Print and shaded views of the part. All mm, measured from the part's lowest x, y and z. A direction names the side the tool comes from. Round coordinates to 2 decimals unless told otherwise and drop trailing zeros. Write each loop counter-clockwise with the first axis right and the second up, starting at its lowest first coordinate (ties: lowest second). Pieces come first, ordered by that corner, then holes. Notation, with made-up numbers: (0.25, 30) - (44.25, 30) arc R19 ccw to (44.25, 59) - close; hole circle Ø9 at (66, 31.25). An arc over 180 degrees is marked (long way). Answer as a JSON object with one key per item and string values. Group by question number.
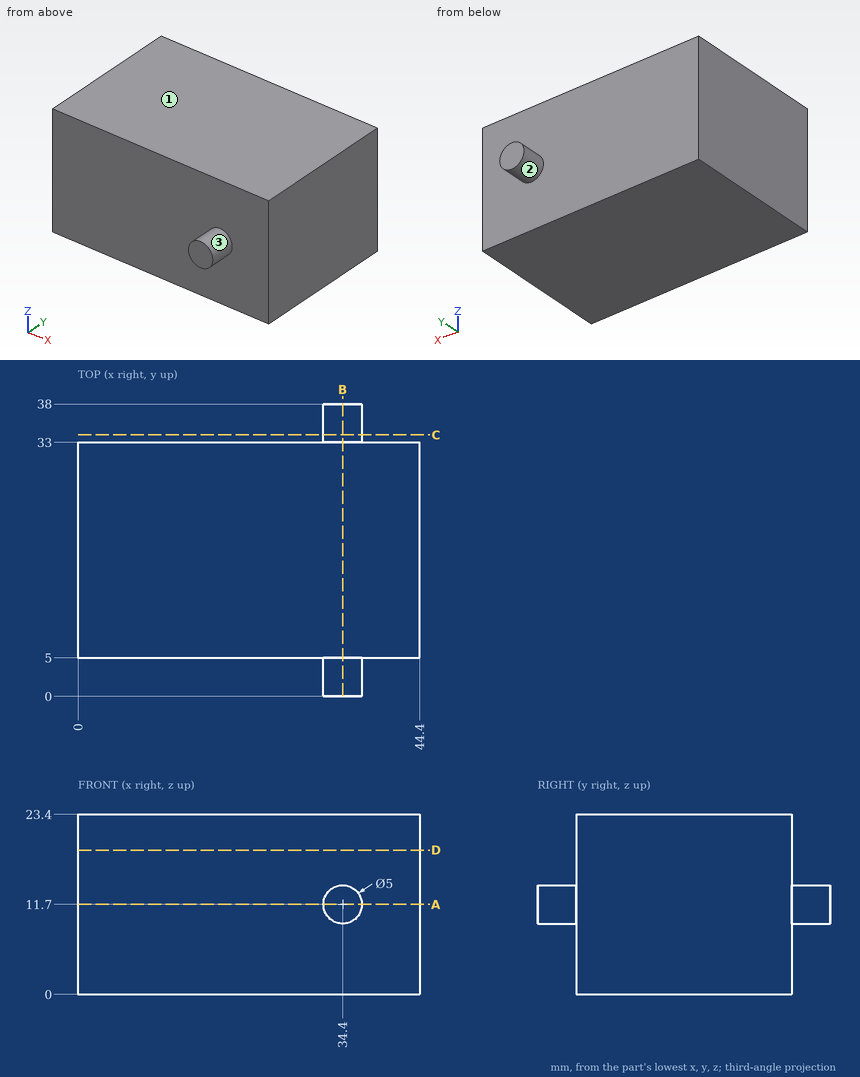
(1) Flat gauge pins, fed straight in: pin 1 (7 mm diameter, centred on x = 11, z = 11, fed in from -Y); pin 2 (6 mm diameter, centred on x = 12.5, z = 9.5, fed in from +Y). Where does each tip first touch, or does it go through?
(2) 3-axis set-ups, long thin cutter, end or side, ignore diameter. For the marked faces 1, 2 and 3: which of +Z, -Z, +X, -X, +Y, -Y reach the whole face in a straight line?
(3) Slice it at D-D (z = 18.75). Write the cut outline in (x, y), then the cut area to 3 significant figures.
(4) Drill centre lines: line 1 (Y direction, x = 20.5, z = 2); line 2 (Z direction, x = 33, y = 36). Where is each one in solid material? Low to high. Write a range as from..to.
(5) Slice it at B-B (x = 34.4). Write the cut outline in (y, z).
(6) Slice it at A-A (z = 11.7). Write the cut outline in (x, y).
(7) Slice it at C-C (y = 34). Write the cut outline in (x, z).
Answer:
{
 "1": {"pin 1": "y = 5", "pin 2": "y = 33"},
 "2": {"face 1": "+Z, +X, -X, +Y, -Y", "face 2": "+Y", "face 3": "-Y"},
 "3": {"outline": "(0, 5) - (44.4, 5) - (44.4, 33) - (0, 33) - close", "area": "1,240 mm²"},
 "4": {"line 1": "5..33", "line 2": "9.63..13.77"},
 "5": {"outline": "(0, 9.2) - (5, 9.2) - (5, 0) - (33, 0) - (33, 9.2) - (38, 9.2) - (38, 14.2) - (33, 14.2) - (33, 23.4) - (5, 23.4) - (5, 14.2) - (0, 14.2) - close"},
 "6": {"outline": "(0, 5) - (31.9, 5) - (31.9, 0) - (36.9, 0) - (36.9, 5) - (44.4, 5) - (44.4, 33) - (36.9, 33) - (36.9, 38) - (31.9, 38) - (31.9, 33) - (0, 33) - close"},
 "7": {"outline": "circle Ø5 at (34.4, 11.7)"}
}
